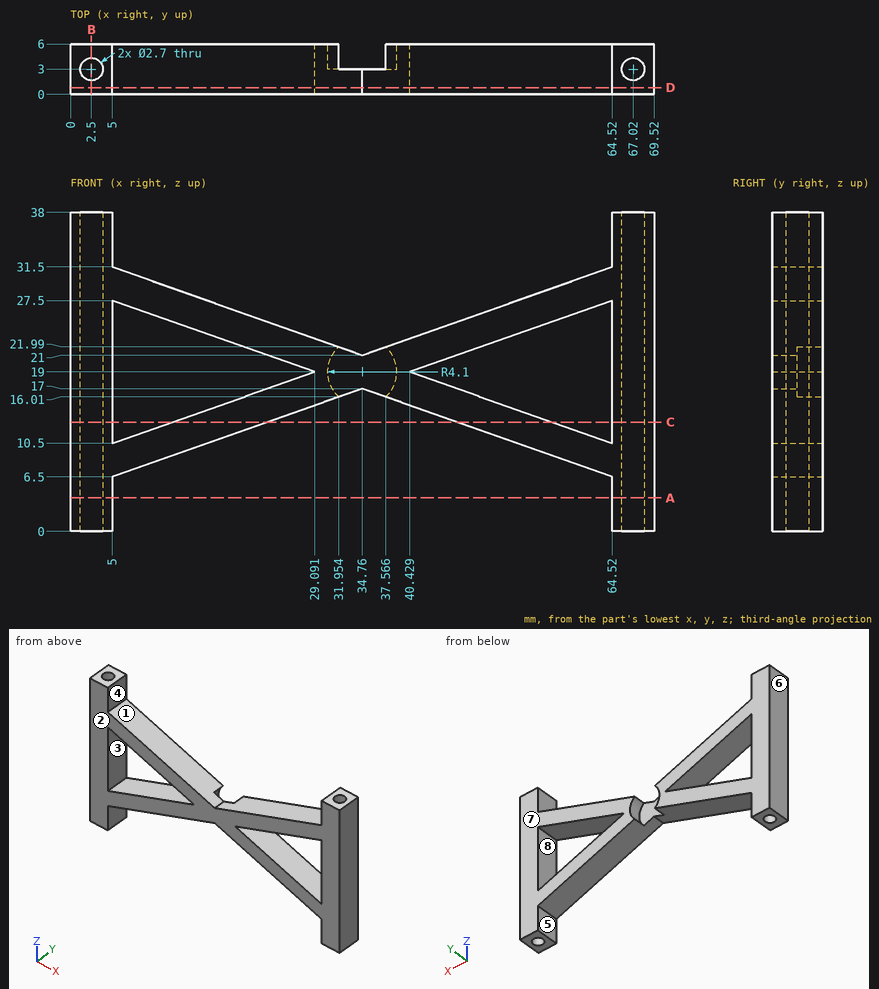
For this review, use the dimensioned drawing (mm, ordinates from the lowest corner) and the shaded views. A direction names the side the tool comes from. Round coordinates to 2 decimals unless told otherwise and drop trailing zeros. Loops run counter-clockwise (first coordinate to the right, second up) from the corner with the lowest first, then second, coordinate; pieces in that order, holes last. Notation, with made-up numbers: (47, 64.25) -> (56, 64.25) arc R18 ccw to (56, 76.25) -> close; hole circle Ø4 at (35.5, 84). An arc over 180 degrees is marked (long way). Write item = value, one per line. Start each with the question number.
Item 1: To check wall thickness, follow L1, parallel to X at y = 3.15, z = 2.5; L2, parallel to Y at x = 67.02, z = 20.5; L3, parallel to X at y = 4.75, z = 6. State the ranges of each line that lie inside material, in increasing order.
Item 2: Take a section at B-B on x = 2.5. Give the boundary of the cut face in (y, z).
Item 3: Take a section at C-C on z = 13. Count the separate pieces of the cut face and the enclosed holes in it.
Item 4: Mouldability with a two-part tool opening along Z and no side actions: class the marked faces 1, 2 and 3 as released by +Z, released by -Z, zero draft, split by the parting line, or undercut.
Item 5: Take a section at D-D on y = 0.8. Give the boundary of the cut face in (x, z).
Item 6: Insertion check: pin 1 (3 mm diameter, centred on x = 33, z = 20.5, fed in from +Y); pin 2 (1 mm diameter, centred on x = 21, y = 1, fed in from -Z). Each pin has a flat end and moves straight along its axis. Give the tip position at first contact, or say it passes through.
Item 7: Take a section at A-A on z = 4. Give the boundary of the cut face in (x, y).
Item 8: For the marked faces 4, 5, 6, 7 and 8, list the 3-axis set-ups (+Z, -Z, +X, -X, +Y, -Y) from which the entire face can be reached by the end or side of a thin tool; tool diameter is ignored.
Result:
q1.L1 = 0 to 1.16, 3.84 to 5, 64.52 to 65.68, 68.36 to 69.52
q1.L2 = 0 to 1.65, 4.35 to 6
q1.L3 = 0 to 5, 64.52 to 69.52
q2.outline = (0, 0) -> (1.65, 0) -> (1.65, 38) -> (0, 38) -> close; (4.35, 0) -> (6, 0) -> (6, 38) -> (4.35, 38) -> close
q3.separate_pieces = 4
q3.enclosed_holes = 2
q4.face_1 = released by +Z
q4.face_2 = zero draft
q4.face_3 = undercut
q5.outline = (0, 0) -> (5, 0) -> (5, 6.5) -> (34.76, 17) -> (64.52, 6.5) -> (64.52, 0) -> (69.52, 0) -> (69.52, 38) -> (64.52, 38) -> (64.52, 31.5) -> (34.76, 21) -> (5, 31.5) -> (5, 38) -> (0, 38) -> close; hole (5, 10.5) -> (29.09, 19) -> (5, 27.5) -> close; hole (40.43, 19) -> (64.52, 10.5) -> (64.52, 27.5) -> close
q6.pin_1 = 3
q6.pin_2 = 11.97
q7.outline = (0, 0) -> (5, 0) -> (5, 6) -> (0, 6) -> close; (64.52, 0) -> (69.52, 0) -> (69.52, 6) -> (64.52, 6) -> close; hole circle Ø2.7 at (2.5, 3); hole circle Ø2.7 at (67.02, 3)
q8.face_4 = +Z, +Y, -Y
q8.face_5 = -Z, +Y, -Y
q8.face_6 = +Z, -Z, -X, +Y, -Y
q8.face_7 = +Z, -Z, +X, -X, +Y
q8.face_8 = +Y, -Y
